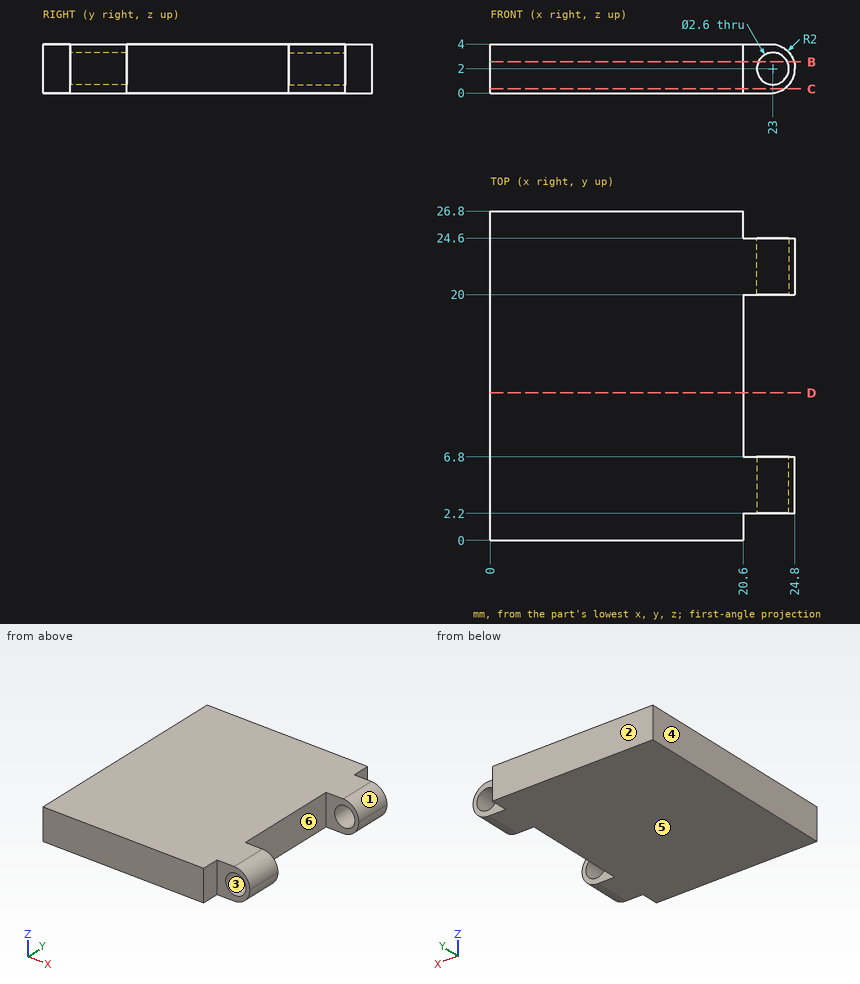
Geometry check sheet. Reference: drawing and pictorial views, mm from the part's lowest x, y, z. A direction names the side the tool comes from. Round coordinates to 2 decimals unless told otherwise and drop trailing zeros. Order: outer loops, then holes, each group sorted by start corner. A loop starts at its lowest first (then second) coordinate and runs counter-clockwise, first axis right, second up. Notation, with made-up numbers: M -4,56.25 L 10,56.25 A14 ccw 10,72.25 Z; hole C 77.25,49 d4. An arc over 180 degrees is marked long. Write item = value, one per line.
Q1. Section check D-D (y = 12). Enter the section's corners in (x, z).
Answer block:
outline = M 0,0 L 20.6,0 L 20.6,4 L 0,4 Z
Q2. Section check B-B (z = 2.55). Enter the section's corners in (x, y), plus the area to 3 significant figures.
Answer block:
outline = M 0,0 L 20.6,0 L 20.6,2.2 L 21.82,2.2 L 21.82,6.8 L 20.6,6.8 L 20.6,20 L 21.82,20 L 21.82,24.6 L 20.6,24.6 L 20.6,26.8 L 0,26.8 Z; M 24.18,2.2 L 24.72,2.2 L 24.72,6.8 L 24.18,6.8 Z; M 24.18,20 L 24.72,20 L 24.72,24.6 L 24.18,24.6 Z
area = 568 mm^2
Q3. Scan lines: line 1 (Y direction, x = 21.25, z = 3.55); line 2 (X direction, y = 1.5, z = 2.6); line 3 (Z direction, x = 23, y = 20.75). Record each from-to range of solid material in increasing order.
Answer block:
line_1 = 2.2 to 6.8, 20 to 24.6
line_2 = 0 to 20.6
line_3 = 0.01 to 0.7, 3.3 to 3.99
Q4. Set-up check for the marked faces 5 and 6: record each of +Z, -Z, +X, -X, +Y, -Y from which the full face is reachable in a straight line by a thin tool's end or side.
Answer block:
face_5 = -Z, +X, -X, +Y, -Y
face_6 = +Z, -Z, +X
Q5. Section check C-C (z = 0.35). Enter the section's corners in (x, y).
Answer block:
outline = M 0,0 L 20.6,0 L 20.6,2.2 L 23.93,2.2 L 23.93,6.8 L 20.6,6.8 L 20.6,20 L 23.93,20 L 23.93,24.6 L 20.6,24.6 L 20.6,26.8 L 0,26.8 Z
Q6. Depth check by flat-ended pin: pin 1 Ø1.8 at (y, z) = (1, 1) entering from +X; pin 2 Ø2 at (x, z) = (23, 2.5) entering from +Y; pin 3 Ø2 at (x, z) = (23.5, 2.5) entering from -Y; pin 4 Ø5 at (x, y) = (21, 16) entering from +Z. Enter the tip coordinate at first touch or a pass-through.
Answer block:
pin_1 = 20.6
pin_2 = 24.6
pin_3 = 2.2
pin_4 = 4
Q7. Release check for a two-part mould opening along X. For the marked faces 1, 2, 3 and 4 record: released by +X, released by -X, zero draft, split by the parting line, or undercut.
Answer block:
face_1 = released by +X
face_2 = zero draft
face_3 = undercut
face_4 = released by -X
